The listing builds one solid part. Answer for the finished solid, in the listing's coordinates (mm). Coordinates: 2 decimals unless noted, no trailing zeros. Order: outer loops, then holes, each group sorted by start corner. A loop starts at its lowest first (then second) coordinate and runs counter-clockwise, first axis right, second up. Notation, with made-up numbers: (51.5, -1.75) -> (108.5, -1.75) arc R22 cw to (108.5, 34.25) -> close; hole circle Ø7 at (59.5, 13). An arc over 180 degrees is marked (long way). Answer in a Markdown table with one row per item. Add a question column.
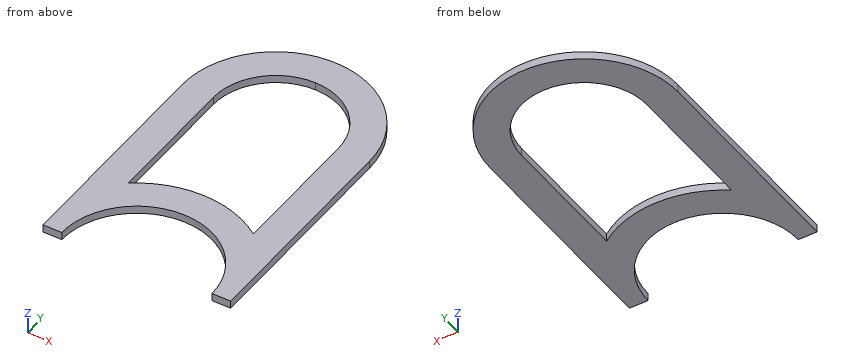
```python
from build123d import *

# Parameters (mm, degrees)
F1_DEPTH = 25


with BuildPart() as f1:
    # F0 (on Top) → F1 (new body)
    with BuildSketch(Plane.XY):
        with BuildLine():
            Line((-255.484788, 651.733869), (-255.484788, -48.266131))
            Line((-255.484788, -48.266131), (-195.484788, -48.266131))
            ThreePointArc((-195.484788, -48.266131), (44.515212, 191.733869), (284.515212, -48.266131))
            Line((284.515212, -48.266131), (344.515212, -48.266131))
            Line((344.515212, -48.266131), (344.515212, 441.456646))
            Line((344.515212, 441.456646), (344.515212, 651.733869))
            ThreePointArc((344.515212, 651.733869), (44.515212, 951.733869), (-255.484788, 651.733869))
        make_face()
        with BuildLine():
            Line((-155.484788, 223.761452), (-155.484788, 651.733869))
            ThreePointArc((-155.484788, 651.733869), (-96.906144, 793.155225), (44.515212, 851.733869))
            ThreePointArc((44.515212, 851.733869), (185.936568, 793.155225), (244.515212, 651.733869))
            Line((244.515212, 651.733869), (244.515212, 223.761452))
            ThreePointArc((244.515212, 223.761452), (44.515212, 288.806911), (-155.484788, 223.761452))
        make_face(mode=Mode.SUBTRACT)
    extrude(amount=F1_DEPTH)


solid = f1.part
```
Q1. A cutting plane is placed at A-A (y = 334.5). Determine the outline of the cut face in (x, z).
Q2. Given pin 1 (4 mm diameter, centred on y = 833, z = 3, fed in from -X); pin 2 (3 mm diameter, centred on x = 262, z = 9, fed in from -Y); pin 3 (4 mm diameter, centred on x = 253.5, z = 5.5, fed in from +Y), each flat-ended and moving along its own axis, determine where each tip first touches the part or whether it passes through.
Q3. A cutting plane is placed at D-D (x = 295). Determine the outline of the cut face in (y, z), then the cut area to 3 significant figures.
Q4. A cutting plane is placed at C-C (x = 100). Determine the outline of the cut face in (y, z).
Q5. Straight lines are drawn through the part: line 1 (X direction, y = 313.5, z = 15.5); line 2 (Y direction, x = 41, z = 1.75); line 3 (X direction, y = 773, z = 11.5). For each, find the intervals that lie inside material, in ascending order.
Q6. A cutting plane is placed at B-B (z = 19.25). Determine the outline of the cut face in (x, y).
Returned:
| question | item | result |
|---|---|---|
| 1 | outline | (-255.48, 0) -> (-155.48, 0) -> (-155.48, 25) -> (-255.48, 25) -> close; (244.52, 0) -> (344.52, 0) -> (344.52, 25) -> (244.52, 25) -> close |
| 2 | pin 1 | stops at x = -196.03 |
| 2 | pin 2 | stops at y = 49.95 |
| 2 | pin 3 | stops at y = 868.89 |
| 3 | outline | (-48.27, 0) -> (816.83, 0) -> (816.83, 25) -> (-48.27, 25) -> close |
| 3 | area | 21,600 mm² |
| 4 | outline | (185.23, 0) -> (284.25, 0) -> (284.25, 25) -> (185.23, 25) -> close; (843.88, 0) -> (946.56, 0) -> (946.56, 25) -> (843.88, 25) -> close |
| 5 | line 1 | x = -255.48 to -155.48, 244.52 to 344.52 |
| 5 | line 2 | y = 191.71 to 288.79, 851.7 to 951.71 |
| 5 | line 3 | x = -229.88 to -114.53, 203.56 to 318.91 |
| 6 | outline | (-255.48, -48.27) -> (-195.48, -48.27) arc R240 cw to (284.52, -48.27) -> (344.52, -48.27) -> (344.52, 651.73) arc R300 ccw to (-255.48, 651.73) -> close; hole (-155.48, 223.76) arc R340 cw to (244.52, 223.76) -> (244.52, 651.73) arc R200 ccw to (44.52, 851.73) arc R200 ccw to (-155.48, 651.73) -> close |
